from build123d import *

# Parameters (mm, degrees)
F0_R     = 4
F0_R_2   = 2.6
F1_DEPTH = 15
F2_R     = 2
F3_W     = 13
F3_H     = 9
F4_DEPTH = 5


with BuildPart() as f1:
    # F0 (on Front) → F1 (new body)
    with BuildSketch(Plane.XZ):
        with BuildLine():
            Line((20.75, 22), (-20.75, 22))
            Line((-20.75, 22), (-20.75, 6.062178))
            ThreePointArc((-20.75, 6.062178), (-17.25, 0), (-20.75, -6.062178))
            Line((-20.75, -6.062178), (-20.75, -18))
            Line((-20.75, -18), (20.75, -18))
            Line((20.75, -18), (20.75, -6.062178))
            ThreePointArc((20.75, -6.062178), (17.25, 0), (20.75, 6.062178))
            Line((20.75, 6.062178), (20.75, 22))
        make_face()
        with Locations((-13.75, -11)):
            Circle(F0_R, mode=Mode.SUBTRACT)
        with Locations((0, -8.5)):
            Circle(F0_R_2, mode=Mode.SUBTRACT)
        with Locations((13.75, -11)):
            Circle(F0_R, mode=Mode.SUBTRACT)
        with Locations((-13.75, 15)):
            Circle(F0_R, mode=Mode.SUBTRACT)
        with Locations((0, 11.5)):
            Circle(F0_R_2, mode=Mode.SUBTRACT)
        with Locations((13.75, 15)):
            Circle(F0_R, mode=Mode.SUBTRACT)
    extrude(amount=F1_DEPTH)

    # F2
    f2_edges = [f1.edges().sort_by_distance(p)[0] for p in [
        (-20.75, -7.5, 22),
        (20.75, -7.5, 22),
        (-20.75, -7.5, -18),
        (20.75, -7.5, -18),
        (20.75, -7.5, 6.062178),
        (20.75, -7.5, -6.062178),
        (-20.75, -7.5, 6.062178),
        (-20.75, -7.5, -6.062178),
    ]]
    fillet(f2_edges, radius=F2_R)

    # F3 (on face) → F4 (join)
    with BuildSketch(Plane.XZ.offset(15)):
        with Locations((0, 2)):
            Rectangle(F3_W, F3_H)
    extrude(amount=F4_DEPTH)


solid = f1.part
The listing builds one solid part. Answer for the finished solid, in the listing's coordinates (mm). A direction names the side the tool comes from. Coordinates: 2 decimals unless noted, no trailing zeros. Write each loop counter-clockwise with the first axis right and the second up, starting at its lowest first coordinate (ties: lowest second). Pieces come first, ordered by that corner, then holes. Notation, with made-up numbers: M 47,70.25 L 87,70.25 A12 cw 87,74.25 Z; hole C 70.5,68.5 d9. An arc over 180 degrees is marked long. Use one line per item in the form item = value.
Item 1: Given P1, Ø1, axis at x = 3, z = -13, coming from the -Y side; P2, Ø1.5, axis at y = -18.5, z = 4, coming from the -X side; P3, Ø6, axis at y = -6, z = 1, coming from the +X side, each flat-ended and moving along its own axis, determine where each tip first touches the part or whether it passes through.
Model answer:
P1 = -15
P2 = -6.5
P3 = 18.51
Item 2: Find section B-B, the plane y = -4.75. Give the vertices of the cut face in (x, z), plus the area to 3 significant figures.
Model answer:
outline = M -20.75,-16 A2 ccw -18.75,-18 L 18.75,-18 A2 ccw 20.75,-16 L 20.75,-7.12 A2 ccw 19.97,-5.54 A7 cw 19.97,5.54 A2 ccw 20.75,7.12 L 20.75,20 A2 ccw 18.75,22 L -18.75,22 A2 ccw -20.75,20 L -20.75,7.12 A2 ccw -19.97,5.54 A7 cw -19.97,-5.54 A2 ccw -20.75,-7.12 Z; hole C -13.75,-11 d8; hole C -13.75,15 d8; hole C 0,-8.5 d5.2; hole C 0,11.5 d5.2; hole C 13.75,-11 d8; hole C 13.75,15 d8
area = 1,350 mm2
Item 3: Find section D-D, the plane x = -4.5. Give the vertices of the cut face in (y, z), plus the area to 3 significant figures.
Model answer:
outline = M -20,-2.5 L -15,-2.5 L -15,-18 L 0,-18 L 0,22 L -15,22 L -15,6.5 L -20,6.5 Z
area = 645 mm2
Item 4: For faces 5 (the face through (0, -17, -2.5)), 6 (the face through (6.5, -17, 2)), 7 (the face through (-20.15, -7.6, 21.43)), 8 (the face through (-20.54, -7.6, -6.23)), determine the directions among +Z, -Z, +X, -X, +Y, -Y from which every point of the face is accessible in a straight line to the end or side of a thin tool.
Model answer:
face_5 = -Z, +X, -X, -Y
face_6 = +Z, -Z, +X, -Y
face_7 = +Z, -X, +Y, -Y
face_8 = -X, +Y, -Y
Item 5: Find section A-A, the plane x = 0. Give the vertices of the cut face in (y, z).
Model answer:
outline = M -20,-2.5 L -15,-2.5 L -15,-5.9 L 0,-5.9 L 0,8.9 L -15,8.9 L -15,6.5 L -20,6.5 Z; M -15,-18 L 0,-18 L 0,-11.1 L -15,-11.1 Z; M -15,14.1 L 0,14.1 L 0,22 L -15,22 Z
Item 6: Find section C-C, the plane z = 15. Give the vertices of the cut face in (x, y), plus the area to 4 significant figures.
Model answer:
outline = M -20.75,-15 L -17.75,-15 L -17.75,0 L -20.75,0 Z; M -9.75,-15 L 9.75,-15 L 9.75,0 L -9.75,0 Z; M 17.75,-15 L 20.75,-15 L 20.75,0 L 17.75,0 Z
area = 382.5 mm2
Item 7: Find the intervals of material crossed by probe 1 along Z at (x, y) = (0, -10.5); probe 2 along Z at (x, y) = (13.75, -11.75); probe 3 along X at (y, z) = (-11, 14.5), in increasing order.
Model answer:
probe_1 = -18 to -11.1, -5.9 to 8.9, 14.1 to 22
probe_2 = -18 to -15, -7 to 11, 19 to 22
probe_3 = -20.75 to -17.72, -9.78 to 9.78, 17.72 to 20.75
Item 8: The mould has two halves that part along X. Classify faces 1 (the face through (-6.5, -17, 2)), 2 (the face through (0, -17, 6.5)), 3 (the face through (-0.56, -7.4, 8.96)), 4 (the face through (-0.56, -7.4, -11.04)): released by +X, released by -X, zero draft, split by the parting line, or undercut.
Model answer:
face_1 = released by -X
face_2 = zero draft
face_3 = undercut
face_4 = undercut
